Here's how the part is built. I have some questions about the finished solid (model axes, mm). A direction names the side the tool comes from. Give positions to 0.01 mm unless a question says otherwise; leave off trailing zeros. Write each loop counter-clockwise with the first axis right and the second up, starting at its lowest first coordinate (ties: lowest second). Pieces come first, ordered by that corner, then holes. Notation, with made-up numbers: (-14, -38) - (34, -38) arc R18 ccw to (34, -15) - close; hole circle Ø1 at (-26.5, 88). An arc over 180 degrees is marked (long way). One line per item, written item: value. Start each with the question number.
1) Imagine slicing it at D-D on x = 97. Write out the boundary of the cut face in (y, z).
2) Imagine slicing it at B-B on x = -125. Write out the boundary of the cut face in (y, z).
3) Imagine slicing it at C-C on y = 15. Write out the boundary of the cut face in (x, z).
4) On a 3-axis mill with a long thin cutter (end or side, diameter ignored), from which of +Z, -Z, +X, -X, +Y, -Y can I reach the whole of each face in a straight line? I mean faces 4 (the flat face through (-179, 20, 0)), 5 (the flat face through (179, 20, 0)), 6 (the flat face through (-3, 35, -5)), 7 (the flat face through (-3, 35, 5)). Say none if no direction works.
5) I'm going to push flat-ended pins straight in: P1, Ø8, axis at y = 19, z = 0.5, coming from the -X side; P2, Ø10, axis at x = 19, z = 42.5, coming from the +Y side; P3, Ø15, axis at x = -14, y = 31.5, coming from the -Z side. Where does each tip first touch, or does it pass through?
6) Imagine slicing it at A-A on z = 0. Write out the boundary of the cut face in (x, y).
7) We'd pull the mould along X, two halves only. Please class faces 1 (the flat face through (-149, 45, 0)), 2 (the flat face through (-3, 5, -55)), 3 (the cylindrical face through (249.326, 4.93, -2.669)): +X half, -X half, draft (parallel to the pull), parting line (faces both ways), or undercut.
8) Please list where these lines run through material, in increasing order: L1, parallel to X at y = 6.25, z = 0; L2, parallel to Y at x = 187, z = 31; L3, parallel to Z at x = -77, y = 29. Write a range as [from, to].
from build123d import *

# Parameters (mm, degrees)
SKETCH_4_R          = 20.5
EXTRUDE_4_DEPTH     = 10
SKETCH_5_W          = 358
SKETCH_5_H          = 10
EXTRUDE_5_DEPTH     = 50
CUT_EXTRUDE_1_DEPTH = 297.405128161


with BuildPart() as part:
    # 草图4 → 凸台-拉伸4 (new body)
    with BuildSketch(Plane(origin=(0, 0, 0), x_dir=(1, 0, 0), z_dir=(0, 1, 0))):
        with BuildLine():
            Line((-229, 55), (229, 55))
            ThreePointArc((229, 55), (284, 0), (229, -55))
            Line((229, -55), (-229, -55))
            ThreePointArc((-229, -55), (-284, 0), (-229, 55))
        make_face()
        with Locations(Location((-229, 0, 0), (0, 0, 270))):
            Circle(SKETCH_4_R, mode=Mode.SUBTRACT)
        with Locations(Location((229, 0, 0), (0, 0, 270))):
            Circle(SKETCH_4_R, mode=Mode.SUBTRACT)
    extrude(amount=EXTRUDE_4_DEPTH)

    # 草图5 → 凸台-拉伸5 (add)
    with BuildSketch(Plane(origin=(0, 10, 0), x_dir=(1, 0, 0), z_dir=(0, 1, 0))):
        Rectangle(SKETCH_5_W, SKETCH_5_H)
    extrude(amount=EXTRUDE_5_DEPTH)

    # 草图6 → 切除-拉伸1 (cut, through all)
    with BuildSketch(Plane.XY.offset(5)):
        Polygon((-179, 60), (-179, 30), (-119, 60), align=None)
        Polygon((179, 60), (179, 30), (119, 60), align=None)
    extrude(amount=-CUT_EXTRUDE_1_DEPTH, mode=Mode.SUBTRACT)


solid = part.part
Numbers:
1. outline: (0, -55) - (10, -55) - (10, -5) - (60, -5) - (60, 5) - (10, 5) - (10, 55) - (0, 55) - close
2. outline: (0, -55) - (10, -55) - (10, -5) - (57, -5) - (57, 5) - (10, 5) - (10, 55) - (0, 55) - close
3. outline: (-179, -5) - (179, -5) - (179, 5) - (-179, 5) - close
4. face 4: +Z, -Z, -X, +Y
4. face 5: +Z, -Z, +X, +Y
4. face 6: -Z, +X, -X, +Y
4. face 7: +Z, +X, -X, +Y
5. P1: x = -179
5. P2: y = 10
5. P3: z = -5
6. outline: (-284, 0) - (-249.5, 0) - (-249.5, 10) - (-284, 10) - close; (-208.5, 0) - (208.5, 0) - (208.5, 10) - (179, 10) - (179, 30) - (119, 60) - (-119, 60) - (-179, 30) - (-179, 10) - (-208.5, 10) - close; (249.5, 0) - (284, 0) - (284, 10) - (249.5, 10) - close
7. face 1: -X half
7. face 2: draft
7. face 3: undercut
8. L1: [-284, -249.5], [-208.5, 208.5], [249.5, 284]
8. L2: [0, 10]
8. L3: [-5, 5]
